Check sheet for the modelled part. Datum: model origin and axes. Units: mm. Coordinates: 2 decimals unless noted, no trailing zeros. Write each loop counter-clockwise with the first axis right and the second up, starting at its lowest first coordinate (ties: lowest second). Pieces come first, ordered by that corner, then holes. Notation, with made-up numbers: M -16.75,-22.75 L -0.75,-22.75 A29 cw -0.75,2.25 Z; hole C 11.5,22.5 d10. An arc over 180 degrees is marked long. Answer as CSV lines item,"result".
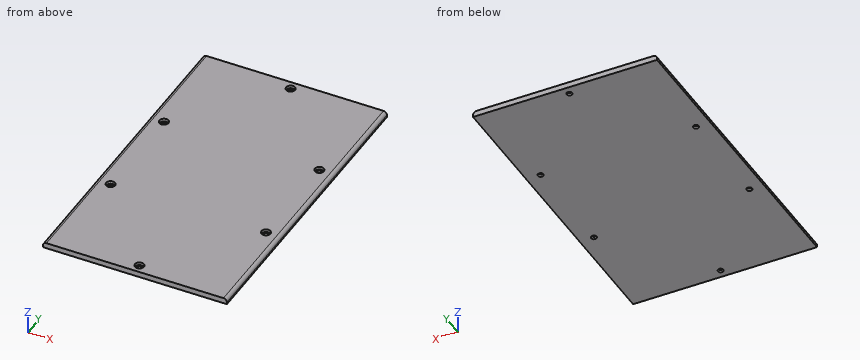
from build123d import *

# Parameters (mm, degrees)
SKETCH_W        = 213
SKETCH_H        = 360
PAD_DEPTH       = 6.5
SKETCH001_R     = 5.2
POCKET_DEPTH    = 3.4
SKETCH002_R     = 3.2
POCKET001_DEPTH = 3.1
FILLET_R        = 4


with BuildPart() as part:
    # Sketch → Pad (new body)
    with BuildSketch(Plane.XY):
        with Locations((106.5, 180)):
            Rectangle(SKETCH_W, SKETCH_H)
    extrude(amount=PAD_DEPTH)

    # Sketch001 (on Face6 of Pad) → Pocket (cut)
    with BuildSketch(Plane.XY.offset(6.5)):
        with Locations((106.5, 350)):
            Circle(SKETCH001_R)
        with Locations((16.5, 240)):
            Circle(SKETCH001_R)
        with Locations((16.5, 120)):
            Circle(SKETCH001_R)
        with Locations((196.5, 240)):
            Circle(SKETCH001_R)
        with Locations((196.5, 120)):
            Circle(SKETCH001_R)
        with Locations((106.5, 10)):
            Circle(SKETCH001_R)
    extrude(amount=-POCKET_DEPTH, mode=Mode.SUBTRACT)

    # Sketch002 (on Face17 of Pocket) → Pocket001 (cut)
    with BuildSketch(Plane.XY.offset(3.1)):
        with Locations((106.5, 350)):
            Circle(SKETCH002_R)
        with Locations((16.5, 240)):
            Circle(SKETCH002_R)
        with Locations((16.5, 120)):
            Circle(SKETCH002_R)
        with Locations((196.5, 240)):
            Circle(SKETCH002_R)
        with Locations((196.5, 120)):
            Circle(SKETCH002_R)
        with Locations((106.5, 10)):
            Circle(SKETCH002_R)
    extrude(amount=-POCKET001_DEPTH, mode=Mode.SUBTRACT)

    # Fillet
    fillet_edges = [part.edges().sort_by_distance(p)[0] for p in [
        (213, 180, 6.5),
        (0, 180, 6.5),
    ]]
    fillet(fillet_edges, radius=FILLET_R)


solid = part.part
1) Depth check by flat-ended pin: P1, Ø10, axis at x = 196.5, y = 120, coming from the +Z side; P2, Ø6, axis at x = 196.5, y = 120, coming from the +Z side; P3, Ø1, axis at y = 255.5, z = 6, coming from the -X side; P4, Ø3, axis at y = 108.5, z = 5.5, coming from the +X side. Enter the tip coordinate at first touch or a pass-through.
Answer key:
P1,"stops at z = 3.1"
P2,"passes through"
P3,"stops at x = 1.35"
P4,"stops at x = 212.71"
2) Section check A-A, the plane z = 5.5. Record the boundary of the cut face in (x, y), plus the area to 3 significant figures.
Answer key:
outline,"M 1.35,0 L 211.65,0 L 211.65,360 L 1.35,360 Z; hole C 16.5,120 d10.4; hole C 16.5,240 d10.4; hole C 106.5,10 d10.4; hole C 106.5,350 d10.4; hole C 196.5,120 d10.4; hole C 196.5,240 d10.4"
area,"75,200 mm2"
3) Thickness scan on line 1 along Y through (x, z) = (16.5, 2.35); line 2 along Y through (x, z) = (106.5, 4.75); line 3 along X through (y, z) = (330, 2.75). Record the ranges inside material, lowest first.
Answer key:
line 1,"y = 0 to 116.8, 123.2 to 236.8, 243.2 to 360"
line 2,"y = 0 to 4.8, 15.2 to 344.8, 355.2 to 360"
line 3,"x = 0.01 to 212.99"
